Build history of the part. All positions in model axes, mm. A direction names the side the tool comes from. Round coordinates to 2 decimals unless told otherwise and drop trailing zeros. Write each loop counter-clockwise with the first axis right and the second up, starting at its lowest first coordinate (ties: lowest second). Pieces come first, ordered by that corner, then holes. Notation, with made-up numbers: M -16,40.5 L 1,40.5 A31 ccw 1,68.5 Z; hole C 41.5,71.25 d1. An arc over 180 degrees is marked long. Write item = value, one per line.
from build123d import *

# Parameters (mm, degrees)
F1_DEPTH = 76.2
F3_DEPTH = 12.701
F5_DEPTH = 101.601


with BuildPart() as f1:
    # F0 (on Front) → F1 (new body)
    with BuildSketch(Plane.XZ):
        Polygon((0, 12.7), (0, 0), (38.1, 0), (38.1, 19.05), (88.9, 19.05), (88.9, 0), (127, 0), (127, 12.7), (101.6, 12.7), (101.6, 50.8), (25.4, 50.8), (25.4, 12.7), align=None)
    extrude(amount=F1_DEPTH)

    # F2 (on face) → F3 (cut, through all)
    with BuildSketch(Plane.XY.offset(12.7)):
        Polygon((101.6, -50.8), (127, -76.2), (127, 0), (101.6, -25.4), align=None)
    extrude(amount=-F3_DEPTH, mode=Mode.SUBTRACT)

    # F4 (on face) → F5 (cut, through all)
    with BuildSketch(Plane.YZ.offset(101.6)):
        Polygon((-25.4, 50.8), (-50.8, 50.8), (-38.1, 38.1), align=None)
    extrude(amount=-F5_DEPTH, mode=Mode.SUBTRACT)


solid = f1.part
1. Band-saw the part on D-D (z = 47). List the corners of the cut face in (x, y).
Responses:
outline = M 25.4,-76.2 L 101.6,-76.2 L 101.6,-47 L 25.4,-47 Z; M 25.4,-29.2 L 101.6,-29.2 L 101.6,0 L 25.4,0 Z
2. Mould opens along X. For faces 4 (the face through (88.9, -38, 10)), 5 (the face through (109, -69, 12.7)), 6 (the face through (38.1, -38, 9)), 7 (the face through (114.1, -63.3, 6.4)) say: pulls with the +X half, pulls with the -X half, needs draft (parallel to the pull), parting line crosses it, or undercut.
Responses:
face_4 = undercut
face_5 = needs draft
face_6 = undercut
face_7 = pulls with the +X half
3. Probe probe 1 along X at (y, z) = (-26, 15); probe 2 along Z at (x, y) = (60, -58); probe 3 along X at (y, z) = (-10, 20). List the from-to ranges inside material, lowest first.
Responses:
probe_1 = 25.4 to 38.1, 88.9 to 101.6
probe_2 = 19.05 to 50.8
probe_3 = 25.4 to 101.6
4. Band-saw the part on A-A (z = 7). List the corners of the cut face in (x, y).
Responses:
outline = M 0,-76.2 L 38.1,-76.2 L 38.1,0 L 0,0 Z; M 88.9,-76.2 L 127,-76.2 L 101.6,-50.8 L 101.6,-25.4 L 127,0 L 88.9,0 Z
5. Tool access for faces 1 (the face through (63, -38, 19.05)), 2 (the face through (109, -7, 12.7)), 3 (the face through (64, -45, 45)): list every direction of +Z, -Z, +X, -X, +Y, -Y with a clear straight run to the whole face (end or side of a thin tool).
Responses:
face_1 = -Z, +Y, -Y
face_2 = +Z, +X, +Y, -Y
face_3 = +Z, +X, -X
6. Band-saw the part on C-C (y = -59). List the corners of the cut face in (x, z), plus the area to 3 significant figures.
Responses:
outline = M 0,0 L 38.1,0 L 38.1,19.05 L 88.9,19.05 L 88.9,0 L 109.8,0 L 109.8,12.7 L 101.6,12.7 L 101.6,50.8 L 25.4,50.8 L 25.4,12.7 L 0,12.7 Z
area = 3,330 mm²
7. Flat gauge pins, fed straight in: pin 1 (15 mm diameter, centred on y = -37.5, z = 27, fed in from +X); pin 2 (12.5 mm diameter, centred on x = 120, y = -65, fed in from +Z); pin 3 (12 mm diameter, centred on x = 60, y = -44.5, fed in from +Z). Where does each tip first touch, or does it go through?
Responses:
pin_1 = 101.6
pin_2 = 12.7
pin_3 = 50.5
8. Band-saw the part on B-B (x = 74). List the corners of the cut face in (y, z).
Responses:
outline = M -76.2,19.05 L 0,19.05 L 0,50.8 L -25.4,50.8 L -38.1,38.1 L -50.8,50.8 L -76.2,50.8 Z
